Read the model definition and answer for the solid it produces. Units are mm, in the model's axes. Round coordinates to 2 decimals unless told otherwise and drop trailing zeros. Write each loop counter-clockwise with the first axis right and the second up, starting at its lowest first coordinate (ties: lowest second). Pieces come first, ordered by that corner, then holes. Notation, with made-up numbers: (-7.75, 89.5) - (35.25, 89.5) arc R30 ccw to (35.25, 127.5) - close; hole circle Ø8 at (81, 27.5). An arc over 180 degrees is marked (long way). Use one line per item in the form item = value. Start each with the question number.
1) The part is cut by section A-A, the plane x = -9.25. Give the vertices of the cut face in (y, z), plus the area to 3 significant figures.
2) The part is cut by section C-C, the plane x = 0. Give the vertices of the cut face in (y, z), plus the area to 3 significant figures.
3) Consider line 1 along X through (y, z) = (-0.55, -0.75); line 2 along Z through (x, y) = (-4.75, -0.4); line 3 along Z through (x, y) = (0, -0.75). Determine where each line is inside the solid, lowest interval first. Write a range as from..to.
4) This flat-tipped pin is pushed along its axis until it touches: pin 1 (1.8 mm diameter, centred on x = 5, z = 8.76, fed in from -Y). Where does it stop, or does it pass through?
5) The part is cut by section B-B, the plane y = -0.95. Count the separate pieces of the cut face and the enclosed holes in it, plus the area to 3 significant figures.
6) For a pull along X with two mould halves and no side action, classify faces 1 (the face through (3.997, -0.592, -8.719)), 2 (the face through (-8.717, -0.592, -8.536)), 3 (the face through (0, 0, 0)) as released by +X, released by -X, zero draft, split by the parting line, or undercut.
7) The part is cut by section D-D, the plane z = -6.75. Give the vertices of the cut face in (x, y), plus the area to 3 significant figures.
from build123d import *

# Parameters (mm, degrees)
F0_R     = 1
F1_DEPTH = 1.2


with BuildPart() as f1:
    # F0 (on Front) → F1 (new body)
    with BuildSketch(Plane.XZ):
        with BuildLine():
            ThreePointArc((12.1915929204, -0.4528377904), (10.3, 0), (12.1915929204, 0.4528377904))
            ThreePointArc((12.1915929204, 0.4528377904), (8.6267027305, 8.6267027305), (0.4528377904, 12.1915929204))
            ThreePointArc((0.4528377904, 12.1915929204), (0.852302115, 11.823049811), (1, 11.3))
            ThreePointArc((1, 11.3), (-0.523049811, 10.447697885), (-0.4528377904, 12.1915929204))
            ThreePointArc((-0.4528377904, 12.1915929204), (-8.6267027305, 8.6267027305), (-12.1915929204, 0.4528377904))
            ThreePointArc((-12.1915929204, 0.4528377904), (-11.0671834632, 0.9725206734), (-10.3, 0))
            ThreePointArc((-10.3, 0), (-11.0671834632, -0.9725206734), (-12.1915929204, -0.4528377904))
            ThreePointArc((-12.1915929204, -0.4528377904), (-8.6267027305, -8.6267027305), (-0.4528377904, -12.1915929204))
            ThreePointArc((-0.4528377904, -12.1915929204), (-0.523049811, -10.447697885), (1, -11.3))
            ThreePointArc((1, -11.3), (0.852302115, -11.823049811), (0.4528377904, -12.1915929204))
            ThreePointArc((0.4528377904, -12.1915929204), (8.6267027305, -8.6267027305), (12.1915929204, -0.4528377904))
        make_face()
        with Locations((-4.996208501, -8.7626928542)):
            Circle(F0_R, mode=Mode.SUBTRACT)
        with Locations((-8.7629663243, -4.9959350308)):
            Circle(F0_R, mode=Mode.SUBTRACT)
        with Locations((4.9959350308, -8.7629663243)):
            Circle(F0_R, mode=Mode.SUBTRACT)
        with Locations((8.7626928542, -4.996208501)):
            Circle(F0_R, mode=Mode.SUBTRACT)
        with Locations((-8.7626928542, 4.996208501)):
            Circle(F0_R, mode=Mode.SUBTRACT)
        with Locations((-4.9959350308, 8.7629663243)):
            Circle(F0_R, mode=Mode.SUBTRACT)
        with Locations((8.7629663243, 4.9959350308)):
            Circle(F0_R, mode=Mode.SUBTRACT)
        with Locations((4.996208501, 8.7626928542)):
            Circle(F0_R, mode=Mode.SUBTRACT)
    extrude(amount=F1_DEPTH)


solid = f1.part
Geometry results:
q1.outline = (-1.2, -7.95) - (0, -7.95) - (0, -5.87) - (-1.2, -5.87) - close; (-1.2, -4.12) - (0, -4.12) - (0, 4.12) - (-1.2, 4.12) - close; (-1.2, 5.87) - (0, 5.87) - (0, 7.95) - (-1.2, 7.95) - close
q1.area = 14.9 mm2
q2.outline = (-1.2, -10.3) - (0, -10.3) - (0, 10.3) - (-1.2, 10.3) - close
q2.area = 24.7 mm2
q3.line_1 = -12.18..-11.96, -10.64..10.64, 11.96..12.18
q3.line_2 = -11.24..-9.73, -7.79..7.79, 9.73..11.24
q3.line_3 = -10.3..10.3
q4.pin_1 = through
q5.separate_pieces = 1
q5.enclosed_holes = 8
q5.area = 430 mm2
q6.face_1 = undercut
q6.face_2 = released by -X
q6.face_3 = zero draft
q7.outline = (-10.16, -1.2) - (10.16, -1.2) - (10.16, 0) - (-10.16, 0) - close
q7.area = 24.4 mm2
